The listing builds one solid part. Answer for the finished solid, in the listing's coordinates (mm). A direction names the side the tool comes from. Coordinates: 2 decimals unless noted, no trailing zeros. Loops run counter-clockwise (first coordinate to the right, second up) from the corner with the lowest first, then second, coordinate; pieces in that order, holes last. Notation, with made-up numbers: (-4.75, 36.5) - (17.25, 36.5) arc R12 cw to (17.25, 48.5) - close; hole circle Ø10 at (-25.75, 86.5). An arc over 180 degrees is marked (long way). Use one line per item in the form item = value. Start each with the question number.
```python
from build123d import *

# Parameters (mm, degrees)
SKETCH_1_W          = 35.5
SKETCH_1_H          = 17.6
SKETCH_1_R          = 1.5
EXTRUDE_1_DEPTH     = 38
CUT_EXTRUDE_1_DEPTH = 39
SKETCH_4_W          = 29.5
SKETCH_4_H          = 28
CUT_EXTRUDE_3_DEPTH = 18.6
SKETCH_5_W          = 35.5
SKETCH_5_H          = 33
CUT_EXTRUDE_4_DEPTH = 18.6
CHAMFER_1_SIZE      = 3
SKETCH_7_R          = 1.25
CUT_EXTRUDE_5_DEPTH = 18.6


with BuildPart() as part:
    # 草图1 → 凸台-拉伸1 (new body)
    with BuildSketch(Plane(origin=(0, 0, 0), x_dir=(1, 0, 0), z_dir=(0, 1, 0))):
        Rectangle(SKETCH_1_W, SKETCH_1_H)
        with Locations((-14, 5)):
            Circle(SKETCH_1_R, mode=Mode.SUBTRACT)
        with Locations((-14, -5)):
            Circle(SKETCH_1_R, mode=Mode.SUBTRACT)
        with Locations((14, -5)):
            Circle(SKETCH_1_R, mode=Mode.SUBTRACT)
        with Locations((14, 5)):
            Circle(SKETCH_1_R, mode=Mode.SUBTRACT)
    extrude(amount=EXTRUDE_1_DEPTH)

    # 草图2 → 切除-拉伸1 (cut, through all)
    with BuildSketch(Plane(origin=(0, 38, 0), x_dir=(1, 0, 0), z_dir=(0, 1, 0))):
        with BuildLine():
            Line((9.7, 5.8), (-9.7, 5.8))
            ThreePointArc((-9.7, 5.8), (-10.265685425, 5.565685425), (-10.5, 5))
            ThreePointArc((-10.5, 5), (-11.525126266, 2.525126266), (-14, 1.5))
            Line((-14, 1.5), (-14.75, 1.5))
            ThreePointArc((-14.75, 1.5), (-15.457106781, 1.207106781), (-15.75, 0.5))
            Line((-15.75, 0.5), (-15.75, -0.5))
            ThreePointArc((-15.75, -0.5), (-15.457106781, -1.207106781), (-14.75, -1.5))
            Line((-14.75, -1.5), (-14, -1.5))
            ThreePointArc((-14, -1.5), (-11.525126266, -2.525126266), (-10.5, -5))
            ThreePointArc((-10.5, -5), (-10.265685425, -5.565685425), (-9.7, -5.8))
            Line((-9.7, -5.8), (9.7, -5.8))
            ThreePointArc((9.7, -5.8), (10.265685425, -5.565685425), (10.5, -5))
            ThreePointArc((10.5, -5), (11.525126266, -2.525126266), (14, -1.5))
            Line((14, -1.5), (14.75, -1.5))
            ThreePointArc((14.75, -1.5), (15.457106781, -1.207106781), (15.75, -0.5))
            Line((15.75, -0.5), (15.75, 0.5))
            ThreePointArc((15.75, 0.5), (15.457106781, 1.207106781), (14.75, 1.5))
            Line((14.75, 1.5), (14, 1.5))
            ThreePointArc((14, 1.5), (11.525126266, 2.525126266), (10.5, 5))
            ThreePointArc((10.5, 5), (10.265685425, 5.565685425), (9.7, 5.8))
        make_face()
    extrude(amount=-CUT_EXTRUDE_1_DEPTH, mode=Mode.SUBTRACT)

    # 草图4 → 切除-拉伸3 (cut, through all)
    with BuildSketch(Plane.XY.offset(8.8)):
        with Locations((0, 19)):
            Rectangle(SKETCH_4_W, SKETCH_4_H)
    extrude(amount=-CUT_EXTRUDE_3_DEPTH, mode=Mode.SUBTRACT)

    # 草图5 → 切除-拉伸4 (cut, through all)
    with BuildSketch(Plane.XY.offset(8.8)):
        with Locations((0, 16.5)):
            Rectangle(SKETCH_5_W, SKETCH_5_H)
    extrude(amount=-CUT_EXTRUDE_4_DEPTH, mode=Mode.SUBTRACT)

    # 倒角1
    chamfer_1_edges = [part.edges().sort_by_distance(p)[0] for p in [
        (17.75, 35.5, 8.8),
        (-17.75, 35.5, 8.8),
        (-17.75, 35.5, -8.8),
        (17.75, 35.5, -8.8),
    ]]
    chamfer(chamfer_1_edges, length=CHAMFER_1_SIZE)

    # 草图7 → 切除-拉伸5 (cut, through all)
    with BuildSketch(Plane(origin=(0, 0, -8.8), x_dir=(-1, 0, 0), z_dir=(0, 0, -1))):
        with Locations((-8.5, 35.5)):
            Circle(SKETCH_7_R)
        with Locations((8.5, 35.5)):
            Circle(SKETCH_7_R)
    extrude(amount=-CUT_EXTRUDE_5_DEPTH, mode=Mode.SUBTRACT)


solid = part.part
```
(1) A cutting plane is placed at D-D (y = 35.5). State how many separate pieces and enclosed holes the cut face has, then the cut area to 3 significant figures.
(2) This flat-tipped pin is pushed along its axis until it touches: pin 1 Ø1.8 at (x, z) = (-14, 5) entering from -Y. Where does it stop, or does it pass through?
(3) Determine the mould class of faces 3 (the face through (-16.23, 35.47, 7.32)), 4 (the face through (-10.26, 35.53, -5.57)), 5 (the face through (0, 38, -6)) for opening direction Z: +Z half, -Z half, draft (parallel to the pull), parting line (faces both ways), or undercut.
(4) A cutting plane is placed at C-C (x = 3). Determine the outline of the cut face in (y, z).
(5) Find the intervals of material crossed by probe 1 along Z at (x, y) = (-14, 35.9); probe 2 along X at (y, z) = (35.65, -5); probe 3 along Z at (x, y) = (14.5, 34.65), in increasing order. Write a range as from..to.
(6) A cutting plane is placed at B-B (z = 7.25). Determine the outline of the cut face in (x, y).
(7) A cutting plane is placed at A-A (x = -8.5). Determine the outline of the cut face in (y, z), then the cut area to 3 significant figures.
(8) For faces 1 (the face through (0, 36, -5.8)), 2 (the face through (16.23, 35.47, -7.32)), determine the directions among +Z, -Z, +X, -X, +Y, -Y from which every point of the face is accessible in a straight line to the end or side of a thin tool.
Evaluation:
q1.separate_pieces = 4
q1.enclosed_holes = 4
q1.area = 264 mm^2
q2.pin_1 = through
q3.face_3 = +Z half
q3.face_4 = undercut
q3.face_5 = draft
q4.outline = (33, -8.8) - (38, -8.8) - (38, -5.8) - (33, -5.8) - close; (33, 5.8) - (38, 5.8) - (38, 8.8) - (33, 8.8) - close
q5.probe_1 = -8.8..-6.5, -3.5..-1.5, 1.5..3.5, 6.5..8.8
q5.probe_2 = -17.75..-15.5, -12.5..-10.5, 10.5..12.5, 15.5..17.75
q5.probe_3 = -8.8..-6.41, -3.59..-1.5, 1.5..3.59, 6.41..8.8
q6.outline = (-16.3, 33) - (16.3, 33) - (16.3, 38) - (-16.3, 38) - close; hole circle Ø2.5 at (-8.5, 35.5); hole circle Ø2.5 at (8.5, 35.5)
q7.outline = (33, -8.8) - (34.25, -8.8) - (34.25, -5.8) - (33, -5.8) - close; (33, 5.8) - (34.25, 5.8) - (34.25, 8.8) - (33, 8.8) - close; (36.75, -8.8) - (38, -8.8) - (38, -5.8) - (36.75, -5.8) - close; (36.75, 5.8) - (38, 5.8) - (38, 8.8) - (36.75, 8.8) - close
q7.area = 15.0 mm^2
q8.face_1 = +Y, -Y
q8.face_2 = -Z, +X, +Y, -Y
